Job drawing, mm, ordinate dimensions from the low corner. One solid piece. A direction names the side the tool comes from. Give positions to 0.01 mm unless a question says otherwise; leave off trailing zeros. Write each loop counter-clockwise with the first axis right and the second up, starting at its lowest first coordinate (ties: lowest second). Pieces come first, ordered by that corner, then holes. Notation, with made-up numbers: (-27, 31.5) - (16, 31.5) arc R20 ccw to (16, 54.5) - close; hole circle Ø1 at (40, 50.25). An arc over 180 degrees is marked (long way). Answer in a Markdown table with one row per item. Add a question column.
1. Which spindle directions (+Z, -Z, +X, -X, +Y, -Y) get a long thin tool onto all of the face, cutting with end or side? Do the marked faces 1 and 2. Say none if no direction does.
2. Drop flat-ended pins along their axis: pin 1 Ø3 at (x, y) = (3.5, 3) entering from +Z; pin 2 Ø3 at (x, z) = (5.5, 5) entering from -Y; pin 3 Ø3 at (y, z) = (5.5, 4) entering from +X; pin 4 Ø2 at (x, z) = (7.5, 1) entering from -Y. Give the stop position or say it passes through.
3. Probe line 1 along X through (y, z) = (5.75, 4.5); line 2 along Y through (x, z) = (1.25, 1.75); line 3 along Z through (x, y) = (3, 2.5). List the from-to ranges inside material, lowest first.
4. Pull direction X, two halves, no side cores. Call the marked faces 3, 4 and 5: released by +X, released by -X, zero draft, split by the parting line, or undercut.
5. Band-saw the part on B-B on x = 4.5. Write the cut outline in (y, z), plus the area to 3 significant figures.
6. Band-saw the part on C-C on y = 8.75. Write the cut outline in (x, z).
7. Band-saw the part on A-A on z = 4.5. Write the cut outline in (x, y), plus the area to 3 significant figures.
8. Band-saw the part on D-D on z = 1. Write the cut outline in (x, y), plus the area to 3 significant figures.
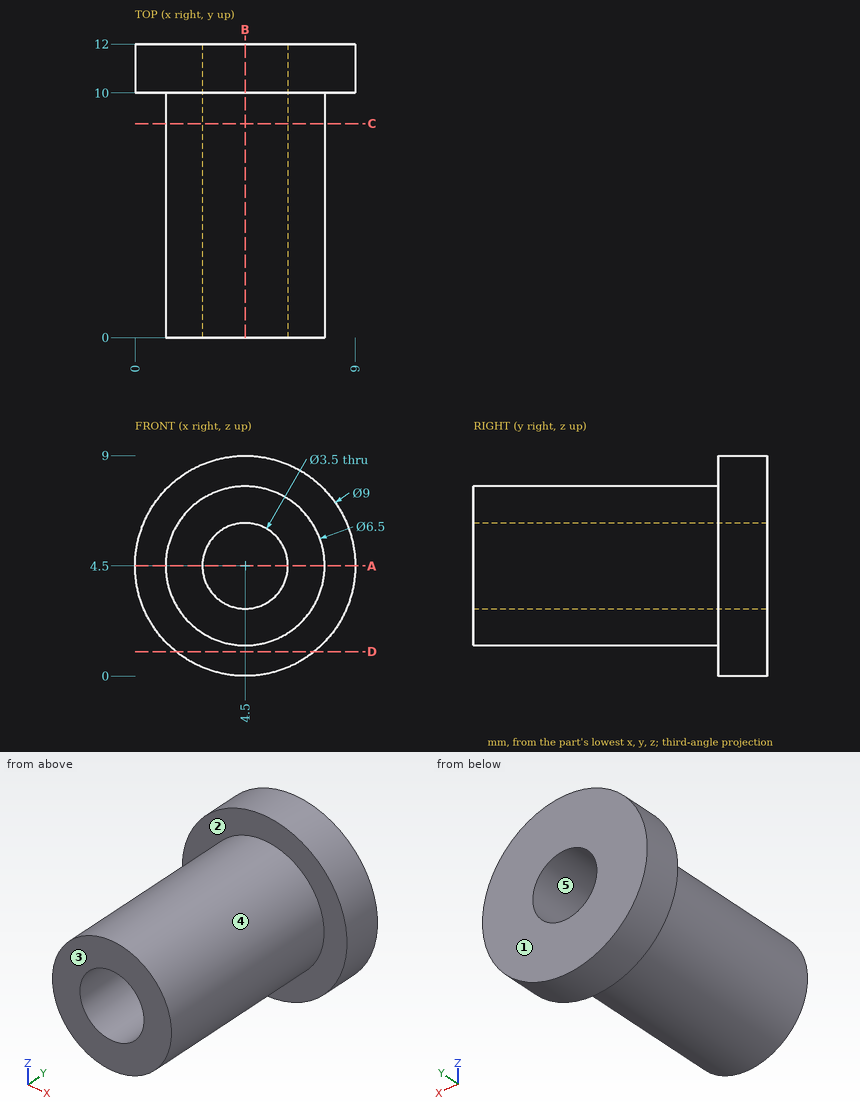
Values:
| question | item | result |
|---|---|---|
| 1 | face 1 | +Z, -Z, +X, -X, +Y |
| 1 | face 2 | -Y |
| 2 | pin 1 | stops at z = 7.75 |
| 2 | pin 2 | stops at y = 0 |
| 2 | pin 3 | stops at x = 7.75 |
| 2 | pin 4 | stops at y = 10 |
| 3 | line 1 | x = 1.25 to 2.75, 6.25 to 7.75 |
| 3 | line 2 | y = 10 to 12 |
| 3 | line 3 | z = 1.62 to 3.6, 5.4 to 7.38 |
| 4 | face 3 | zero draft |
| 4 | face 4 | split by the parting line |
| 4 | face 5 | undercut |
| 5 | outline | (0, 1.25) - (10, 1.25) - (10, 0) - (12, 0) - (12, 2.75) - (0, 2.75) - close; (0, 6.25) - (12, 6.25) - (12, 9) - (10, 9) - (10, 7.75) - (0, 7.75) - close |
| 5 | area | 41.0 mm² |
| 6 | outline | circle Ø6.5 at (4.5, 4.5); hole circle Ø3.5 at (4.5, 4.5) |
| 7 | outline | (0, 10) - (1.25, 10) - (1.25, 0) - (2.75, 0) - (2.75, 12) - (0, 12) - close; (6.25, 0) - (7.75, 0) - (7.75, 10) - (9, 10) - (9, 12) - (6.25, 12) - close |
| 7 | area | 41.0 mm² |
| 8 | outline | (1.67, 10) - (7.33, 10) - (7.33, 12) - (1.67, 12) - close |
| 8 | area | 11.3 mm² |
